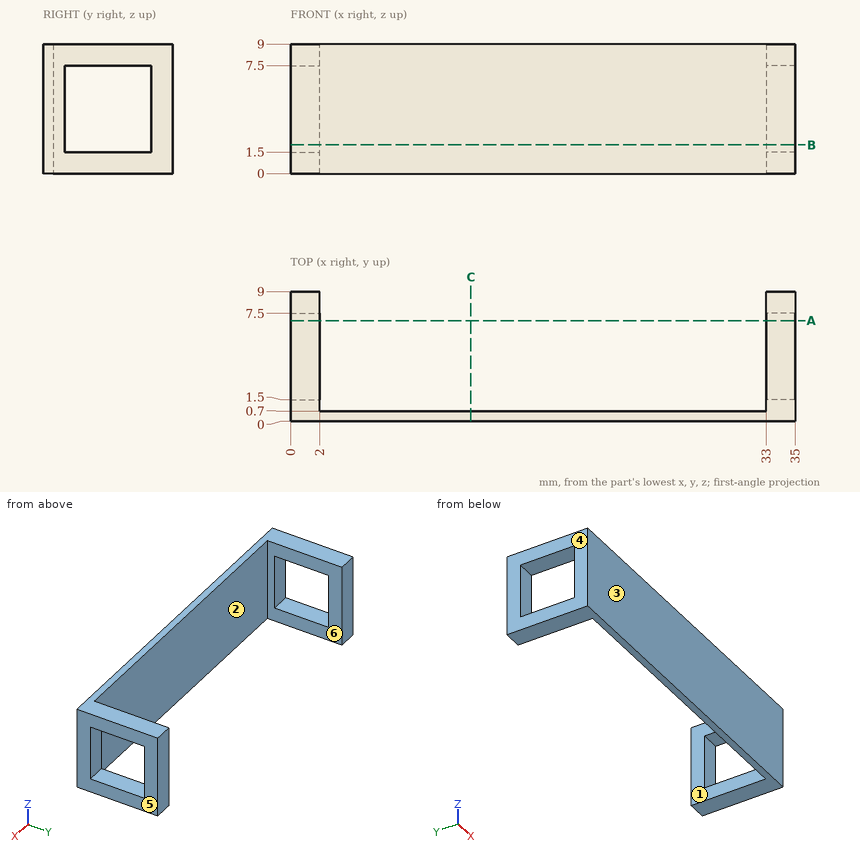
Source: three-view drawing plus pictorial views. Frame: mm from the lowest corner of the part. A direction names the side the tool comes from. Round coordinates to 2 decimals unless told otherwise and drop trailing zeros. Loops run counter-clockwise (first coordinate to the right, second up) from the corner with the lowest first, then second, coordinate; pieces in that order, holes last.
1. Section query B-B on z = 2. Output: boundary loops of the cut face in (x, y).
2. Ray query, L1, parallel to X at y = 1.25, z = 4; L2, parallel to Z at x = 1, y = 2; L3, parallel to Y at x = 30, z = 5.25. Return the intervals inside material, ascending.
3. Section query A-A on y = 7. Output: boundary loops of the cut face in (x, z), and give its area (3 significant figures).
4. Section query C-C on x = 12.5. Output: boundary loops of the cut face in (y, z).
5. Access query for the marked faces 5 and 6. Directions: +Z, -Z, +X, -X, +Y, -Y. A direction counts if a zero-diameter tool reaches every point of the face in a straight line with its end or side. Return the directions, or none.
6. Contact query for a flat-ended pin moving along its axis: pin 1 (1.5 mm diameter, centred on x = 9.5, z = 3.5, fed in from +Y). Output: stop coordinate, or through.
7. Mould query, pull axis X, two halves, no side actions, for the marked faces 1, 2, 3 and 4. Classes: released by +X, released by -X, zero draft, split by the parting line, or undercut.
Answers below:
1. outline: (0, 0) - (35, 0) - (35, 1.5) - (33, 1.5) - (33, 0.7) - (2, 0.7) - (2, 1.5) - (0, 1.5) - close; (0, 7.5) - (2, 7.5) - (2, 9) - (0, 9) - close; (33, 7.5) - (35, 7.5) - (35, 9) - (33, 9) - close
2. L1: x = 0 to 2, 33 to 35
2. L2: z = 0 to 1.5, 7.5 to 9
2. L3: y = 0 to 0.7
3. outline: (0, 0) - (2, 0) - (2, 1.5) - (0, 1.5) - close; (0, 7.5) - (2, 7.5) - (2, 9) - (0, 9) - close; (33, 0) - (35, 0) - (35, 1.5) - (33, 1.5) - close; (33, 7.5) - (35, 7.5) - (35, 9) - (33, 9) - close
3. area: 12.0 mm2
4. outline: (0, 0) - (0.7, 0) - (0.7, 9) - (0, 9) - close
5. face 5: +Z, -Z, +X, +Y, -Y
5. face 6: +Z, -Z, +Y
6. pin 1: stops at y = 0.7
7. face 1: undercut
7. face 2: undercut
7. face 3: zero draft
7. face 4: released by -X
